Build history of the part. All positions in model axes, mm. A direction names the side the tool comes from. Round coordinates to 2 decimals unless told otherwise and drop trailing zeros. Write each loop counter-clockwise with the first axis right and the second up, starting at its lowest first coordinate (ties: lowest second). Pieces come first, ordered by that corner, then holes. Notation, with made-up numbers: (88, -25) - (120, -25) arc R23 cw to (120, -12) - close; hole circle Ø6 at (60.25, 6). An arc over 180 degrees is marked (long way). Write each question's results on one line, items separated by ' | '.
from build123d import *

# Parameters (mm, degrees)
F0_W     = 1200
F0_H     = 450
F1_DEPTH = 250
F2_T     = -5
F3_W     = 5
F3_H     = 142.5
F3_H_2   = 5
F4_DEPTH = 245
F5_R     = 18.5
F6_DEPTH = 25


with BuildPart() as f1:
    # F0 (on Top) → F1 (new body)
    with BuildSketch(Plane.XY):
        Rectangle(F0_W, F0_H)
    extrude(amount=F1_DEPTH)

    # F2
    f2_openings = [f1.faces().sort_by_distance(p)[0] for p in [
        (0, 0, 250),
    ]]
    offset(amount=F2_T, openings=f2_openings)

    # F3 (on face) → F4 (join, through all)
    with BuildSketch(Plane.XY.offset(5)):
        Polygon((302.5, -77.5), (595, -77.5), (595, -72.5), (2.5, -72.5), (-595, -72.5), (-595, -75), (-595, -77.5), (-302.5, -77.5), (-297.5, -77.5), (-2.5, -77.5), (2.5, -77.5), (297.5, -77.5), align=None)
        with Locations((300, -148.75)):
            Rectangle(F3_W, F3_H)
        Polygon((2.5, 72.5), (595, 72.5), (595, 77.5), (302.5, 77.5), (297.5, 77.5), (2.5, 77.5), align=None)
        Polygon((0, -220), (2.5, -220), (2.5, -77.5), (-2.5, -77.5), (-2.5, -220), align=None)
        with Locations((0, 75)):
            Rectangle(F3_W, F3_H_2)
        with Locations((300, 148.75)):
            Rectangle(F3_W, F3_H)
        Polygon((-595, 72.5), (-2.5, 72.5), (-2.5, 77.5), (-297.5, 77.5), (-302.5, 77.5), (-595, 77.5), (-595, 75), align=None)
        with Locations((0, 148.75)):
            Rectangle(F3_W, F3_H)
        Polygon((-297.5, -220), (-297.5, -77.5), (-302.5, -77.5), (-302.5, -220), (-300, -220), align=None)
        with Locations((-300, 148.75)):
            Rectangle(F3_W, F3_H)
    extrude(amount=F4_DEPTH)

    # F5 (on face) → F6 (cut)
    with BuildSketch(Plane.XY.offset(5)):
        with Locations((-42.5, 117.5)):
            Circle(F5_R)
        with Locations((-342.5, 117.5)):
            Circle(F5_R)
        with Locations((-342.5, -117.5)):
            Circle(F5_R)
        with Locations((-42.5, -117.5)):
            Circle(F5_R)
        with Locations((257.5, -117.5)):
            Circle(F5_R)
        with Locations((257.5, 117.5)):
            Circle(F5_R)
        with Locations((555, 117.5)):
            Circle(F5_R)
        with Locations((555, 0)):
            Circle(F5_R)
        with Locations((555, -117.5)):
            Circle(F5_R)
    extrude(amount=-F6_DEPTH, mode=Mode.SUBTRACT)


solid = f1.part
(1) Slice it at D-D, the plane x = 555. Write the cut outline in (y, z).
Worked answers:
outline: (-225, 0) - (-136, 0) - (-136, 5) - (-220, 5) - (-220, 250) - (-225, 250) - close; (-99, 0) - (-18.5, 0) - (-18.5, 5) - (-72.5, 5) - (-72.5, 250) - (-77.5, 250) - (-77.5, 5) - (-99, 5) - close; (18.5, 0) - (99, 0) - (99, 5) - (77.5, 5) - (77.5, 250) - (72.5, 250) - (72.5, 5) - (18.5, 5) - close; (136, 0) - (225, 0) - (225, 250) - (220, 250) - (220, 5) - (136, 5) - close
(2) Two-plate mould, pull along X, no slides. Class faces 1 (the flat face through (297.5, 148, 126)), 2 (the flat face through (595, -1, 126)), 3 (the flat face through (-8, -225, 123)): released by +X, released by -X, zero draft, split by the parting line, or undercut.
Worked answers:
face 1: undercut | face 2: undercut | face 3: zero draft
(3) Tool access for faces 4 (the cylindrical face through (275.146, 123.057, 2.535)), 5 (the flat face through (-2.5, 148, 126)): list every direction of +Z, -Z, +X, -X, +Y, -Y with a clear straight run to the whole face (end or side of a thin tool).
Worked answers:
face 4: +Z, -Z | face 5: +Z
(4) Slice it at A-A, the plane y = 0. Write the cut outline in (x, z).
Worked answers:
outline: (-600, 0) - (536.5, 0) - (536.5, 5) - (-595, 5) - (-595, 250) - (-600, 250) - close; (573.5, 0) - (600, 0) - (600, 250) - (595, 250) - (595, 5) - (573.5, 5) - close
(5) Slice it at C-C, the plane y = 196. Write the cut outline in (x, z).
Worked answers:
outline: (-600, 0) - (600, 0) - (600, 250) - (595, 250) - (595, 5) - (302.5, 5) - (302.5, 250) - (297.5, 250) - (297.5, 5) - (2.5, 5) - (2.5, 250) - (-2.5, 250) - (-2.5, 5) - (-297.5, 5) - (-297.5, 250) - (-302.5, 250) - (-302.5, 5) - (-595, 5) - (-595, 250) - (-600, 250) - close
(6) Flat gauge pin, fed straight in: pin 1 Ø10 at (x, y) = (182.5, 60) entering from +Z. Where does the tip first touch, or does it go through?
Worked answers:
pin 1: stops at z = 5
(7) Drill centre lines: probe 1 along Y at (x, z) = (-42, 1); probe 2 along Y at (x, z) = (-4.5, 137); probe 3 along X at (y, z) = (131.5, 156). Where is each one in solid material? Low to high. Write a range as [from, to].
Worked answers:
probe 1: y = [-225, -135.99], [-99.01, 99.01], [135.99, 225] | probe 2: y = [-225, -220], [-77.5, -72.5], [72.5, 77.5], [220, 225] | probe 3: x = [-600, -595], [-302.5, -297.5], [-2.5, 2.5], [297.5, 302.5], [595, 600]
(8) Slice it at B-B, the plane x = 257.5. Write the cut outline in (y, z), and give its area (3 significant figures).
Worked answers:
outline: (-225, 0) - (-136, 0) - (-136, 5) - (-220, 5) - (-220, 250) - (-225, 250) - close; (-99, 0) - (99, 0) - (99, 5) - (77.5, 5) - (77.5, 250) - (72.5, 250) - (72.5, 5) - (-72.5, 5) - (-72.5, 250) - (-77.5, 250) - (-77.5, 5) - (-99, 5) - close; (136, 0) - (225, 0) - (225, 250) - (220, 250) - (220, 5) - (136, 5) - close | area: 6,780 mm2
